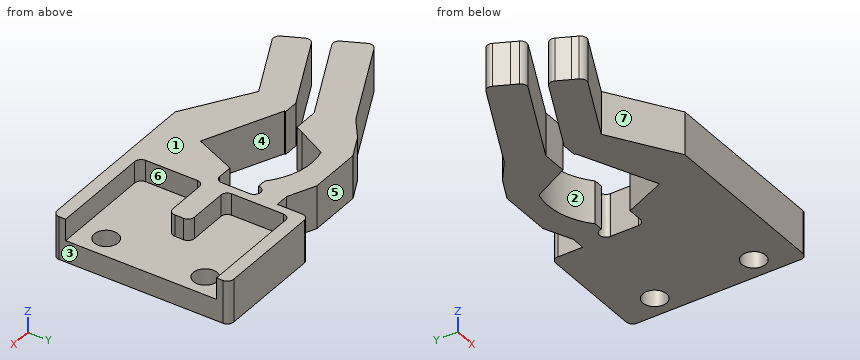
from build123d import *

# Parameters (mm, degrees)
F1_DEPTH = 10
F0_R     = 2.763
F0_R_2   = 2.7634135205
F2_DEPTH = 5


# Not quite as in the source:
# - a feature names something its author has since deleted; it is built from what else it names


with BuildPart() as f1:
    # F0 (on Top) → F1 (new body)
    with BuildSketch(Plane.XY):
        with BuildLine():
            Line((-28.9846330285, 19.3060322961), (-32.4846330285, 19.3060322961))
            Line((-32.4846330285, 19.3060322961), (-36.6950527355, 9.6871775882))
            Line((-36.6950527355, 9.6871775882), (-36.7611596752, 9.5361539153))
            Line((-36.7611596752, 9.5361539153), (-54.1667062895, 17.1550086232))
            Line((-54.1667062895, 17.1550086232), (-54.1667062895, 17.4688580502))
            Line((-54.1667062895, 17.4688580502), (-57.6066188446, 17.4688580502))
            Line((-57.6066188446, 17.4688580502), (-75.9521011029, 8.5636187846))
            ThreePointArc((-75.9521011029, 8.5636187846), (-76.7144296488, 7.7052047395), (-76.6464869407, 6.5591666629))
            Line((-76.6464869407, 6.5591666629), (-75.2652584401, 3.7137290281))
            Line((-75.2652584401, 3.7137290281), (-74.6256538324, 2.3960940233))
            ThreePointArc((-74.6256538324, 2.3960940233), (-73.7672397873, 1.6337654774), (-72.6212017107, 1.7017081855))
            Line((-72.6212017107, 1.7017081855), (-56.8289984312, 9.3675382114))
            Line((-56.8289984312, 9.3675382114), (-42.1148466106, 0))
            Line((-42.1148466106, 0), (-28.5, 0))
            Line((-28.5, 0), (-18.5, 0))
            Line((-18.5, 0), (-1.9846330285, 0))
            ThreePointArc((-1.9846330285, 0), (-0.9239728567, 0.4393398282), (-0.4846330285, 1.5))
            Line((-0.4846330285, 1.5), (-0.4846330285, 3))
            Line((-0.4846330285, 3), (-23.9846330285, 3))
            ThreePointArc((-23.9846330285, 3), (-25.0452932003, 3.4393398282), (-25.4846330285, 4.5))
            Line((-25.4846330285, 4.5), (-25.4846330285, 16.5))
            ThreePointArc((-25.4846330285, 16.5), (-25.0452932003, 17.5606601718), (-23.9846330285, 18))
            Line((-23.9846330285, 18), (-14.9846330285, 18))
            ThreePointArc((-14.9846330285, 18), (-13.9239728567, 18.4393398282), (-13.4846330285, 19.5))
            Line((-13.4846330285, 19.5), (-13.4846330285, 21.5))
            ThreePointArc((-13.4846330285, 21.5), (-13.9239728567, 22.5606601718), (-14.9846330285, 23))
            Line((-14.9846330285, 23), (-23.9846330285, 23))
            ThreePointArc((-23.9846330285, 23), (-25.0452932003, 23.4393398282), (-25.4846330285, 24.5))
            Line((-25.4846330285, 24.5), (-25.4846330285, 36.5))
            ThreePointArc((-25.4846330285, 36.5), (-25.0452932003, 37.5606601718), (-23.9846330285, 38))
            Line((-23.9846330285, 38), (-0.4846330285, 38))
            Line((-0.4846330285, 38), (-0.4846330285, 39.5))
            ThreePointArc((-0.4846330285, 39.5), (-0.9239728567, 40.5606601718), (-1.9846330285, 41))
            Line((-1.9846330285, 41), (-25.4846330285, 41))
            Line((-25.4846330285, 41), (-25.9846330285, 41))
            ThreePointArc((-25.9846330285, 41), (-27.0452932003, 40.5606601718), (-27.4846330285, 39.5))
            Line((-27.4846330285, 39.5), (-27.4846330285, 39.3057436331))
            Line((-27.4846330285, 39.3057436331), (-27.4846330285, 33.7137029542))
            Line((-27.4846330285, 33.7137029542), (-30.6379412534, 33.7137029542))
            Line((-30.6379412534, 33.7137029542), (-36.9315167422, 36.4685625576))
            Line((-36.9315167422, 36.4685625576), (-49.1994071018, 36.4685625576))
            Line((-49.1994071018, 36.4685625576), (-54.7152283086, 33.7718741409))
            Line((-54.7152283086, 33.7718741409), (-59.5651725871, 30.0348878412))
            Line((-59.5651725871, 30.0348878412), (-81.2621656129, 19.502762737))
            ThreePointArc((-81.2621656129, 19.502762737), (-82.0244941588, 18.6443486919), (-81.9565514507, 17.4983106153))
            Line((-81.9565514507, 17.4983106153), (-80.4281407861, 14.3496663292))
            Line((-80.4281407861, 14.3496663292), (-79.683210987, 12.8150532767))
            ThreePointArc((-79.683210987, 12.8150532767), (-78.8247969419, 12.0527247308), (-77.6787588653, 12.1206674389))
            Line((-77.6787588653, 12.1206674389), (-56.8778590157, 22.2178122015))
            Line((-56.8778590157, 22.2178122015), (-51.0782729994, 22.2178122015))
            Line((-51.0782729994, 22.2178122015), (-50.1937510157, 23.9381783364))
            Line((-50.1937510157, 23.9381783364), (-46.6653068671, 30.8008860291))
            ThreePointArc((-46.6653068671, 30.8008860291), (-39.1888505002, 30.8927845811), (-32.6282824459, 27.3060322961))
            Line((-32.6282824459, 27.3060322961), (-30.4846330285, 27.3060322961))
            ThreePointArc((-30.4846330285, 27.3060322961), (-28.9846330285, 28.8060322961), (-27.4846330285, 27.3060322961))
            Line((-27.4846330285, 27.3060322961), (-27.4846330285, 20.8060322961))
            ThreePointArc((-27.4846330285, 20.8060322961), (-27.9239728567, 19.7453721243), (-28.9846330285, 19.3060322961))
        make_face()
    extrude(amount=F1_DEPTH)

    # F0 (on Top) → F2 (join)
    with BuildSketch(Plane.XY):
        with BuildLine():
            Line((-23.9846330285, 3), (-0.4846330285, 3))
            Line((-0.4846330285, 3), (-0.4846330285, 3.0459866499))
            Line((-0.4846330285, 3.0459866499), (-0.4846330285, 37.9540133501))
            Line((-0.4846330285, 37.9540133501), (-0.4846330285, 38))
            Line((-0.4846330285, 38), (-23.9846330285, 38))
            ThreePointArc((-23.9846330285, 38), (-25.0452932003, 37.5606601718), (-25.4846330285, 36.5))
            Line((-25.4846330285, 36.5), (-25.4846330285, 24.5))
            ThreePointArc((-25.4846330285, 24.5), (-25.0452932003, 23.4393398282), (-23.9846330285, 23))
            Line((-23.9846330285, 23), (-14.9846330285, 23))
            ThreePointArc((-14.9846330285, 23), (-13.9239728567, 22.5606601718), (-13.4846330285, 21.5))
            Line((-13.4846330285, 21.5), (-13.4846330285, 19.5))
            ThreePointArc((-13.4846330285, 19.5), (-13.9239728567, 18.4393398282), (-14.9846330285, 18))
            Line((-14.9846330285, 18), (-23.9846330285, 18))
            ThreePointArc((-23.9846330285, 18), (-25.0452932003, 17.5606601718), (-25.4846330285, 16.5))
            Line((-25.4846330285, 16.5), (-25.4846330285, 4.5))
            ThreePointArc((-25.4846330285, 4.5), (-25.0452932003, 3.4393398282), (-23.9846330285, 3))
        make_face()
        with Locations((-5.4846330285, 9)):
            Circle(F0_R, mode=Mode.SUBTRACT)
        with Locations((-5.4846330285, 32)):
            Circle(F0_R_2, mode=Mode.SUBTRACT)
    extrude(amount=F2_DEPTH)


solid = f1.part
Here's how the part is built. I have some questions about the finished solid (model axes, mm). Face numbers are marked on the shaded views. A direction names the side the tool comes from. Give positions to 0.01 mm unless a question says otherwise; leave off trailing zeros. Order: outer loops, then holes, each group sorted by start corner. A loop starts at its lowest first (then second) coordinate and runs counter-clockwise, first axis right, second up. Notation, with made-up numbers: (8.25, -38.5) -> (43.25, -38.5) arc R23 cw to (43.25, 0.5) -> close; hole circle Ø8 at (-5, 76.5). An arc over 180 degrees is marked (long way). Use a Markdown table: item, result. Add a question column.
Item 1: I need wall thicknesses on line 1 (X direction, y = 15.5, z = 4.75); line 2 (Y direction, x = -12, z = 5.75); line 3 (Y direction, x = -33, z = 8.5). Which ranges of each line are inside material? Lowest first, please.
Item 2: If we mould it in two halves opening along X, with no side actions, what happens to the marked faces 1, 2 and 3? For each: pulls with the +X half, pulls with the -X half, needs draft (parallel to the pull), parting line crosses it, or undercut.
Item 3: Imagine slicing it at B-B on x = -6. Please give me the cut outline in (y, z).
Item 4: Imagine slicing it at C-C on z = 4. Give the number of separate pieces and of enclosed holes in the cut face, plus the area to 3 significant figures.
Item 5: Will these pins go through, and if not, where does the flat tip stop? pin 1 (6 mm diameter, centred on x = -64, y = 34, fed in from +Z); pin 2 (3 mm diameter, centred on x = -70, z = 1.5, fed in from -Y); pin 3 (1.5 mm diameter, centred on y = 10, z = 8.5, fed in from +X); pin 4 (4.5 mm diameter, centred on y = 38, z = 3, fed in from -X).
Item 6: For the marked faces 4, 5, 6 and 7, which set-ups out of +Z, -Z, +X, -X, +Y, -Y let a thin tool reach every point of the face, with its end or its side?
Item 7: Imagine slicing it at A-A on x = -40.5. Please give me the cut outline in (y, z), plus the area to 3 significant figures.
Data:
| question | item | result |
|---|---|---|
| 1 | line 1 | x = -80.99 to -70.72, -61.66 to -50.39, -34.15 to -0.48 |
| 1 | line 2 | y = 0 to 3, 38 to 41 |
| 1 | line 3 | y = 0 to 18.13, 27.65 to 34.75 |
| 2 | face 1 | needs draft |
| 2 | face 2 | undercut |
| 2 | face 3 | pulls with the +X half |
| 3 | outline | (0, 0) -> (6.29, 0) -> (6.29, 5) -> (3, 5) -> (3, 10) -> (0, 10) -> close; (11.71, 0) -> (29.29, 0) -> (29.29, 5) -> (11.71, 5) -> close; (34.71, 0) -> (41, 0) -> (41, 10) -> (38, 10) -> (38, 5) -> (34.71, 5) -> close |
| 4 | separate pieces | 1 |
| 4 | enclosed holes | 2 |
| 4 | area | 2,030 mm² |
| 5 | pin 1 | passes through |
| 5 | pin 2 | stops at y = 2.25 |
| 5 | pin 3 | stops at x = -25.48 |
| 5 | pin 4 | stops at x = -50.67 |
| 6 | face 4 | +Z, -Z |
| 6 | face 5 | +Z, -Z, -X, +Y |
| 6 | face 6 | +Z, +X |
| 6 | face 7 | +Z, -Z, -Y |
| 7 | outline | (0, 0) -> (11.17, 0) -> (11.17, 10) -> (0, 10) -> close; (31.16, 0) -> (36.47, 0) -> (36.47, 10) -> (31.16, 10) -> close |
| 7 | area | 165 mm² |
